```python
from build123d import *

# Parameters (mm, degrees)
SKETCH_1_R          = 0.5
EXTRUDE_1_DEPTH     = 2
SKETCH_2_R          = 2.5
CUT_EXTRUDE_1_DEPTH = 1.5
SKETCH_3_R          = 3.75
EXTRUDE_2_DEPTH     = 3
SKETCH_4_R          = 1.3
CUT_EXTRUDE_2_DEPTH = 9
SKETCH_5_R          = 1.3
CUT_EXTRUDE_4_DEPTH = 3


with BuildPart() as part:
    # 草图1 → 凸台-拉伸1 (new body)
    with BuildSketch(Plane.XY):
        with BuildLine():
            Line((0, 3.75), (15.75, 1.5))
            ThreePointArc((15.75, 1.5), (17.25, 0), (15.75, -1.5))
            Line((15.75, -1.5), (0, -3.75))
            ThreePointArc((0, -3.75), (-3.75, 0), (0, 3.75))
        make_face()
        with Locations((14.25, 0)):
            Circle(SKETCH_1_R, mode=Mode.SUBTRACT)
        with Locations((12.25, 0)):
            Circle(SKETCH_1_R, mode=Mode.SUBTRACT)
        with Locations((10.25, 0)):
            Circle(SKETCH_1_R, mode=Mode.SUBTRACT)
        with Locations((8.25, 0)):
            Circle(SKETCH_1_R, mode=Mode.SUBTRACT)
        with Locations((6.25, 0)):
            Circle(SKETCH_1_R, mode=Mode.SUBTRACT)
        with Locations((4.25, 0)):
            Circle(SKETCH_1_R, mode=Mode.SUBTRACT)
    extrude(amount=EXTRUDE_1_DEPTH)

    # 草图2 → 切除-拉伸1 (cut)
    with BuildSketch(Plane(origin=(0, 0, 0), x_dir=(-1, 0, 0), z_dir=(0, 0, -1))):
        Circle(SKETCH_2_R)
    extrude(amount=-CUT_EXTRUDE_1_DEPTH, mode=Mode.SUBTRACT)

    # 草图3 → 凸台-拉伸2 (add)
    with BuildSketch(Plane.XY.offset(2)):
        Circle(SKETCH_3_R)
    extrude(amount=EXTRUDE_2_DEPTH)

    # 草图4 → 切除-拉伸2 (cut)
    with BuildSketch(Plane(origin=(0, 0, 1.5), x_dir=(-1, 0, 0), z_dir=(0, 0, -1))):
        Circle(SKETCH_4_R)
    extrude(amount=-CUT_EXTRUDE_2_DEPTH, mode=Mode.SUBTRACT)

    # 草图5 → 切除-拉伸4 (cut)
    with BuildSketch(Plane.XY.offset(5)):
        Polygon((0, -1.939028966), (0.352599159, -2.491409984), (0.535291858, -1.862065615), (1.02923199, -2.292732659), (1.027217553, -1.637410678), (1.622482567, -1.911473664), (1.435924191, -1.28326436), (2.084289255, -1.378520335), (1.728300791, -0.82831749), (2.377239224, -0.737049382), (1.88066074, -0.309427158), (2.477599408, -0.039028966), (1.88066074, 0.231369227), (2.377239224, 0.658991451), (1.728300791, 0.750259559), (2.084289255, 1.300462404), (1.435924191, 1.205206429), (1.622482567, 1.833415733), (1.027217553, 1.559352747), (1.02923199, 2.214674728), (0.535291858, 1.784007684), (0.352599159, 2.413352053), (0, 1.860971034), (-0.352599159, 2.413352053), (-0.535291858, 1.784007684), (-1.02923199, 2.214674728), (-1.027217553, 1.559352747), (-1.622482567, 1.833415733), (-1.435924191, 1.205206429), (-2.084289255, 1.300462404), (-1.728300791, 0.750259559), (-2.377239224, 0.658991451), (-1.88066074, 0.231369227), (-2.477599408, -0.039028966), (-1.88066074, -0.309427158), (-2.377239224, -0.737049382), (-1.728300791, -0.82831749), (-2.084289255, -1.378520335), (-1.435924191, -1.28326436), (-1.622482567, -1.911473664), (-1.027217553, -1.637410678), (-1.02923199, -2.292732659), (-0.535291858, -1.862065615), (-0.352599159, -2.491409984), align=None)
        Circle(SKETCH_5_R, mode=Mode.SUBTRACT)
    extrude(amount=-CUT_EXTRUDE_4_DEPTH, mode=Mode.SUBTRACT)


solid = part.part
```
The listing builds one solid part. Answer for the finished solid, in the listing's coordinates (mm). A direction names the side the tool comes from. Coordinates: 2 decimals unless noted, no trailing zeros. Loops run counter-clockwise (first coordinate to the right, second up) from the corner with the lowest first, then second, coordinate; pieces in that order, holes last. Notation, with made-up numbers: M -9.75,-24 L 8.25,-24 A10 ccw 8.25,-13 Z; hole C 40,1 d10. An arc over 180 degrees is marked long. Answer as CSV lines item,"result". Start each with the question number.
(1) The part is cut by section A-A (x = 12.25). Give the vertices of the cut face in (y, z), and give its area (3 significant figures).
(2) Find the intervals of material crossed by L1, parallel to Y at x = 0, z = 0.45; L2, parallel to Y at x = 0, z = 1.7; L3, parallel to X at y = -0.25, z = 3.05, in increasing order. Write a range as [from, to].
(3) The part is cut by section B-B (y = -3). Give the vertices of the cut face in (x, z), and give its area (3 significant figures).
(4) Given pin 1 (1.5 mm diameter, centred on y = -1.5, z = 2.5, fed in from -X); pin 2 (3 mm diameter, centred on y = -1, z = 4, fed in from +X); pin 3 (4 mm diameter, centred on x = 13.5, y = 0.5, fed in from +Z), each flat-ended and moving along its own axis, determine where each tip first touches the part or whether it passes through.
(5) The part is cut by section C-C (x = 6.25). Give the vertices of the cut face in (y, z), and give its area (3 significant figures).
(6) The mould has two halves that part along X. Classify faces 1 (the flat face through (2, -2, 5)), 2 (the flat face through (7.99, -2.61, 0.99)), 3 (the cylindrical face through (11.75, 0.02, 0.99)): pulls with the +X half, pulls with the -X half, needs draft (parallel to the pull), parting line crosses it, or undercut.
(7) The part is cut by section D-D (x = 15). Give the vertices of the cut face in (y, z).
(8) For faces 4 (the cylindrical face through (3.85, -0.3, 0.99)), 5 (the flat face through (-1.1, -1.1, 1.5)), determine the directions among +Z, -Z, +X, -X, +Y, -Y from which every point of the face is accessible in a straight line to the end or side of a thin tool.
Determined:
1,outline,"M -2,0 L -0.5,0 L -0.5,2 L -2,2 Z; M 0.5,0 L 2,0 L 2,2 L 0.5,2 Z"
1,area,"6.00 mm2"
2,L1,"[-3.75, -2.5], [2.5, 3.75]"
2,L2,"[-3.75, -1.3], [1.3, 3.75]"
2,L3,"[-3.74, -2.01], [2.01, 3.74]"
3,outline,"M -2.25,0 L 5.25,0 L 5.25,2 L 2.25,2 L 2.25,5 L -2.25,5 Z"
3,area,"28.5 mm2"
4,pin 1,"x = -3.67"
4,pin 2,"x = 3.75"
4,pin 3,"z = 2"
5,outline,"M -2.86,0 L -0.5,0 L -0.5,2 L -2.86,2 Z; M 0.5,0 L 2.86,0 L 2.86,2 L 0.5,2 Z"
5,area,"9.43 mm2"
6,face 1,"needs draft"
6,face 2,"pulls with the +X half"
6,face 3,"undercut"
7,outline,"M -1.61,0 L 1.61,0 L 1.61,2 L -1.61,2 Z"
8,face 4,"+Z, -Z"
8,face 5,"-Z"
